Verification items for the finished model (mm, model axes). Face numbers are marked on the shaded views. A direction names the side the tool comes from. Coordinates: 2 decimals unless noted, no trailing zeros. Loops run counter-clockwise (first coordinate to the right, second up) from the corner with the lowest first, then second, coordinate; pieces in that order, holes last. Notation, with made-up numbers: (49, 39.25) - (100, 39.25) arc R35 cw to (100, 78.25) - close; hole circle Ø6 at (-12, -28). An arc over 180 degrees is marked (long way). Answer as CSV lines item,"result". Start each with the question number.
1. Cross-section at C-C (z = 6.25). Enter the section's corners in (x, y), plus the area to 3 significant figures.
2. Release check for a two-part mould opening along X. For the marked faces 4 and 5 record: pulls with the +X half, pulls with the -X half, needs draft (parallel to the pull), parting line crosses it, or undercut.
3. Material ranges on line 1 (X direction, y = -3.5, z = 1.75); line 2 (Z direction, x = 19, y = -7.5); line 3 (Y direction, x = 9.5, z = 12.5), recorded low to high. Write a range as [from, to].
4. Cross-section at B-B (y = -10). Enter the section's corners in (x, z).
5. Cross-section at A-A (x = 35.5). Enter the section's corners in (y, z), plus the area to 3 significant figures.
6. Set-up check for the marked faces 1, 2 and 3: record each of +Z, -Z, +X, -X, +Y, -Y from which the full face is reachable in a straight line by a thin tool's end or side.
7. Cross-section at D-D (x = 22). Enter the section's corners in (y, z), plus the area to 3 significant figures.
8. Gauge pin test, flat ends, axial feed: P1, Ø0.8, axis at y = -3, z = 3, coming from the +X side; P2, Ø0.8, axis at x = 23, z = 2.5, coming from the +Y side; P3, Ø0.5, axis at y = -3, z = 2.5, coming from the -X side. Record the tip position at first contact, or that the pin passes through.
Autodesk Inventor part; units mm, degrees
ref_plane "YZ Plane" through (0, 0, 0) normal (1, 0, 0) x (0, 1, 0)
ref_plane "XZ Plane" through (0, 0, 0) normal (0, 1, 0) x (-1, 0, 0)
ref_plane "XY Plane" through (0, 0, 0) normal (0, 0, 1) x (1, 0, 0)
sketch "Sketch1" plane through (0, 0, 0) normal (0, 0, 1) x (1, 0, 0)
  line L0 (0, 0) -> (45, 0)
  line L1 (45, 0) -> (45, -20)
  line L2 (45, -20) -> (0, -20)
  line L3 (0, -20) -> (0, 0)
  dimension "d0" = 45
  dimension "d1" = 20
extrude "Extrusion1" add sketch "Sketch1" along normal blind 1
sketch "Sketch2" plane through (0, 0, 1) normal (0, 0, 1) x (1, 0, 0)
  circle A0 centre (9.5, -10) radius 8
  circle A1 centre (35.5, -10) radius 8
  line L0 (0, -20) -> (45, -20)
  line L1 (0, 0) -> (0, -20)
  dimension "d4" = 16
  dimension "d5" = 16
  dimension "d6" = 26
  dimension "d7" = 10
  dimension "d8" = 9.5
extrude "Extrusion2" add sketch "Sketch2" along normal blind 12
sketch "Sketch3" plane through (0, 0, 1) normal (0, 0, 1) x (1, 0, 0)
  line L0 (17.5, -0.5) -> (27.5, -0.5)
  line L1 (27.5, -0.5) -> (27.5, -5.5)
  line L2 (27.5, -5.5) -> (17.5, -5.5)
  line L3 (17.5, -5.5) -> (17.5, -0.5)
  line L4 (0, 0) -> (0, -20)
  line L5 (45, 0) -> (0, 0)
  dimension "d11" = 10
  dimension "d12" = 5
  dimension "d13" = 17.5
  dimension "d14" = 0.5
extrude "Extrusion3" add sketch "Sketch3" along normal blind 3
fillet "Fillet1" radius 2 4 edges at (27.5, -0.5, 2.5) (27.5, -5.5, 2.5) (17.5, -0.5, 2.5) (17.5, -5.5, 2.5)
fillet "Fillet2" radius 0.5 8 edges at (17.5, -3, 4) (18.0858, -1.0858, 4) (22.5, -0.5, 4) (26.9142, -1.0858, 4) (27.5, -3, 4) (26.9142, -4.9142, 4) (22.5, -5.5, 4) (18.0858, -4.9142, 4)
sketch "Sketch4" plane through (0, 0, 0) normal (0, 0, -1) x (-1, 0, 0)
  point P0 (0, 0)
properties part number "UltrasonicSensor"
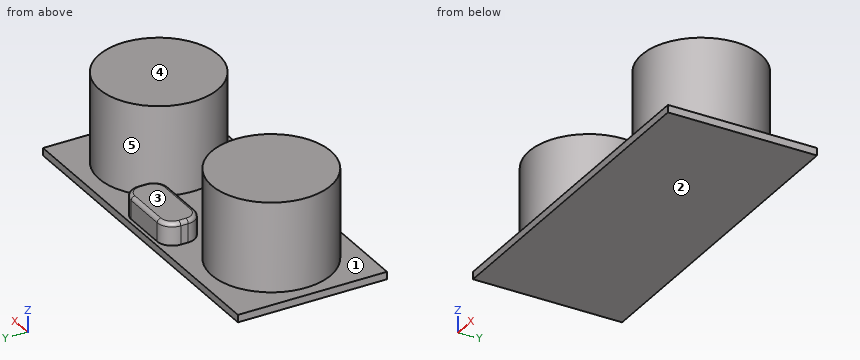
Values follow:
1,outline,"circle Ø16 at (9.5, -10); circle Ø16 at (35.5, -10)"
1,area,"402 mm²"
2,face 4,"needs draft"
2,face 5,"undercut"
3,line 1,"x = [4.84, 14.16], [17.5, 27.5], [30.84, 40.16]"
3,line 2,"z = [0, 1]"
3,line 3,"y = [-18, -2]"
4,outline,"(0, 0) - (45, 0) - (45, 1) - (43.5, 1) - (43.5, 13) - (27.5, 13) - (27.5, 1) - (17.5, 1) - (17.5, 13) - (1.5, 13) - (1.5, 1) - (0, 1) - close"
5,outline,"(-20, 0) - (0, 0) - (0, 1) - (-2, 1) - (-2, 13) - (-18, 13) - (-18, 1) - (-20, 1) - close"
5,area,"212 mm²"
6,face 1,"+Z"
6,face 2,"-Z, +X, -X, +Y, -Y"
6,face 3,"+Z, +Y, -Y"
7,outline,"(-20, 0) - (0, 0) - (0, 1) - (-0.5, 1) - (-0.5, 3.5) arc R0.5 ccw to (-1, 4) - (-5, 4) arc R0.5 ccw to (-5.5, 3.5) - (-5.5, 1) - (-20, 1) - close"
7,area,"34.9 mm²"
8,P1,"stops at x = 40.02"
8,P2,"stops at y = -0.5"
8,P3,"stops at x = 5.21"
